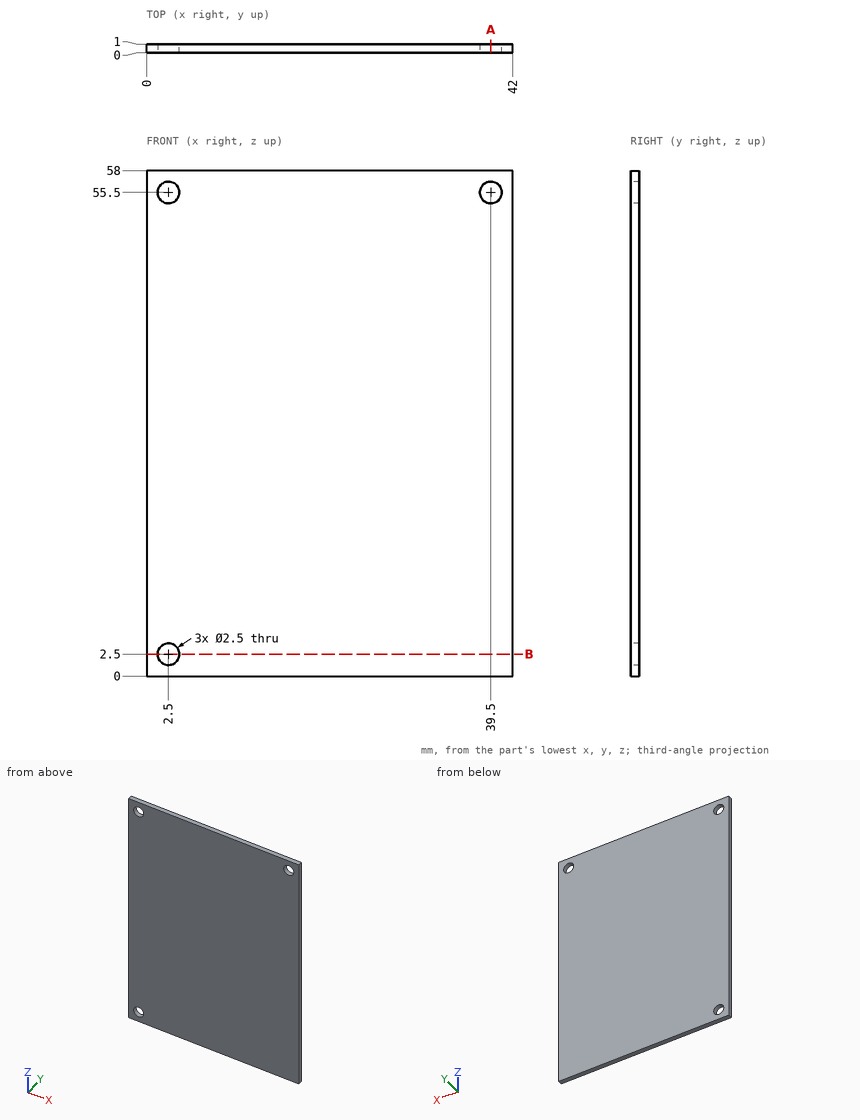
Part print with two shaded views. Sizes in mm from the minimum x, y, z corner. Round coordinates to 2 decimals unless told otherwise and drop trailing zeros. Write each loop counter-clockwise with the first axis right and the second up, starting at its lowest first coordinate (ties: lowest second). Pieces come first, ordered by that corner, then holes. Notation, with made-up numbers: M 82.5,20.25 L 93.5,20.25 A22 ccw 93.5,49.25 Z; hole C 5.5,78 d1. An arc over 180 degrees is marked long. Use CSV: the item, a comma, the result in double quotes.
1. Wall check: probe 1 along Z at (x, y) = (2.5, 0.55); probe 2 along X at (y, z) = (0.6, 55.5); probe 3 along X at (y, z) = (0.35, 2.5). Give the ranges that are in metal, low to high. Write a range as from..to.
Reply:
probe 1,"z = 0..1.25, 3.75..54.25, 56.75..58"
probe 2,"x = 0..1.25, 3.75..38.25, 40.75..42"
probe 3,"x = 0..1.25, 3.75..42"
2. Saw through at B-B (z = 2.5). Give the cut face in (x, y), plus the area to 3 significant figures.
Reply:
outline,"M 0,0 L 1.25,0 L 1.25,1 L 0,1 Z; M 3.75,0 L 42,0 L 42,1 L 3.75,1 Z"
area,"39.5 mm²"
3. Saw through at A-A (x = 39.5). Give the cut face in (y, z), plus the area to 3 significant figures.
Reply:
outline,"M 0,0 L 1,0 L 1,54.25 L 0,54.25 Z; M 0,56.75 L 1,56.75 L 1,58 L 0,58 Z"
area,"55.5 mm²"
